Check sheet for the drawn part. Datum: minimum x, y, z corner. Units: mm. Give positions to 0.01 mm unless a question says otherwise; leave off trailing zeros. Loops run counter-clockwise (first coordinate to the right, second up) from the corner with the lowest first, then second, coordinate; pieces in that order, holes last. Notation, with made-up numbers: (22, -18) - (39, -18) arc R6 cw to (39, -14) - close; hole circle Ø3 at (-18, -39.5). An arc over 180 degrees is marked (long way). One line per item, written item: value. Start each with the question number.
1. Gauge pin test, flat ends, axial feed: pin 1 (2 mm diameter, centred on x = 3, y = 9, fed in from -Z); pin 2 (1.5 mm diameter, centred on y = 9, z = 28, fed in from +X); pin 3 (6 mm diameter, centred on y = 7, z = 34.5, fed in from +X). Record the tip position at first contact, or that the pin passes through.
2. Sectioned sample at B-B (y = 6.35). Record the cut outline in (x, z) (3 decimals), plus the area to 3 significant figures.
3. Sectioned sample at A-A (x = 6.35). Record the cut outline in (y, z) (3 decimals).
4. Sectioned sample at D-D (z = 23.5). Record the cut outline in (x, y).
5. Sectioned sample at C-C (x = 10.5). Record the cut outline in (y, z) (3 decimals).
6. Mould release check, pull along Y, two halves, no side actions. Record for the marked faces 1 and 2: pulls with the +Y half, pulls with the -Y half, needs draft (parallel to the pull), parting line crosses it, or undercut.
7. Scan lines: L1, parallel to X at y = 6.25, z = 81.5; L2, parallel to X at y = 11, z = 35.5. Record each from-to range of solid material in increasing order. Write a range as [from, to].
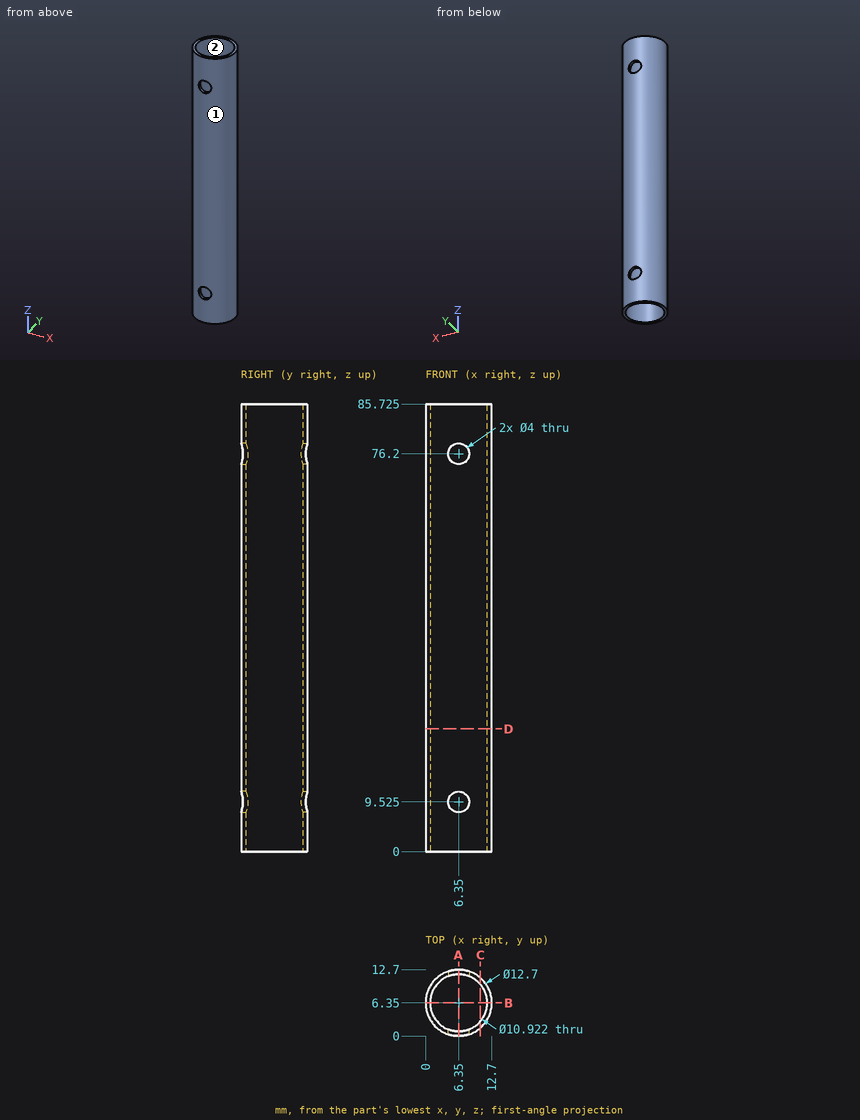
Results are:
1. pin 1: passes through
1. pin 2: stops at x = 12.41
1. pin 3: stops at x = 12.7
2. outline: (0, 0) - (0.889, 0) - (0.889, 85.725) - (0, 85.725) - close; (11.811, 0) - (12.7, 0) - (12.7, 85.725) - (11.811, 85.725) - close
2. area: 152 mm^2
3. outline: (0, 0) - (0.889, 0) - (0.889, 7.525) - (0, 7.525) - close; (0, 11.525) - (0.889, 11.525) - (0.889, 74.2) - (0, 74.2) - close; (0, 78.2) - (0.889, 78.2) - (0.889, 85.725) - (0, 85.725) - close; (11.811, 0) - (12.7, 0) - (12.7, 7.525) - (11.811, 7.525) - close; (11.811, 11.525) - (12.7, 11.525) - (12.7, 74.2) - (11.811, 74.2) - close; (11.811, 78.2) - (12.7, 78.2) - (12.7, 85.725) - (11.811, 85.725) - close
4. outline: circle Ø12.7 at (6.35, 6.35); hole circle Ø10.92 at (6.35, 6.35)
5. outline: (1.544, 0) - (2.8, 0) - (2.8, 85.725) - (1.544, 85.725) - close; (9.9, 0) - (11.156, 0) - (11.156, 85.725) - (9.9, 85.725) - close
6. face 1: parting line crosses it
6. face 2: undercut
7. L1: x = [0, 0.89], [11.81, 12.7]
7. L2: x = [2.03, 3.49], [9.21, 10.67]
